Can you work these out from the model? Positions are in its coordinate system, mm. A direction names the side the tool comes from. Round coordinates to 2 decimals unless told otherwise and drop trailing zeros. Order: outer loops, then holes, each group sorted by start corner. A loop starts at its lowest first (then second) coordinate and runs counter-clockwise, first axis right, second up. Notation, with made-up numbers: (46, -14) -> (61, -14) arc R27 cw to (61, 6) -> close; hole circle Ø2 at (38, 77). An arc over 180 degrees is marked (long way). Use a Markdown table: item, result. Add a question column.
Q1. For faces 1 (the face through (0, 1.25, -10)), 2 (the face through (1.3, -1.5, 1.3)), 3 (the face through (-1.08, -2.96, -4.88)), 4 (the face through (2.5, 2.5, 2.5)), which set-ups out of +Z, -Z, +X, -X, +Y, -Y let a thin tool reach every point of the face, with its end or its side?
Q2. I need wall thicknesses on line 1 along Z through (x, y) = (0, -0.1); line 2 along Y through (x, z) = (9, -4.5); line 3 along X through (y, z) = (-4.5, 1.5). Which ranges of each line are inside material? Lowest first, please. Write a range as [from, to].
Q3. If we section it at D-D on z = 10.75: List the corners of the cut face in (x, y) for me, plus the area to 3 significant figures.
Q4. I'm going to push flat-ended pins straight in: pin 1 Ø3 at (x, z) = (-3, 9.5) entering from -Y; pin 2 Ø1 at (x, z) = (5, -7) entering from -Y; pin 3 Ø8 at (x, z) = (0, 0) entering from -Y; pin 4 Ø2.5 at (x, z) = (0, 0) entering from +Y. Where does each tip first touch, or does it pass through?
Q5. If we section it at C-C on y = -0.75: List the corners of the cut face in (x, z) for me.
Q6. If we section it at A-A on z = 0: List the corners of the cut face in (x, y) for me, plus the area to 3 significant figures.
Q7. If we section it at B-B on y = 1.75: List the corners of the cut face in (x, z) for me.
Q8. We'd pull the mould along Z, two halves only. Please class faces 5 (the face through (0, -4, -2)), 6 (the face through (-0.1, -6, -2.2)), 7 (the face through (10.887, 1.51, -5.046)): +Z half, -Z half, draft (parallel to the pull), parting line (faces both ways), or undercut.
```python
from build123d import *

# Parameters (mm, degrees)
CROQUIS1_R              = 12
SALIENTE_EXTRUIR1_DEPTH = 2.5
CROQUIS3_R              = 5
SALIENTE_EXTRUIR2_DEPTH = 6
CROQUIS2_R              = 3.001453564
CORTAR_EXTRUIR1_DEPTH   = 4
CROQUIS4_R              = 1.5
CORTAR_EXTRUIR2_DEPTH   = 8
CROQUIS5_R              = 2
CORTAR_EXTRUIR6_DEPTH   = 4
CROQUIS6_R              = 1.5
CORTAR_EXTRUIR7_DEPTH   = 4
CROQUIS7_R              = 1
CORTAR_EXTRUIR8_DEPTH   = 4
CORTAR_EXTRUIR9_DEPTH   = 1.25


with BuildPart() as part:
    # Croquis1 → Saliente-Extruir1 (new body)
    with BuildSketch(Plane(origin=(0, 0, 0), x_dir=(1, 0, 0), z_dir=(0, 1, 0))):
        Circle(CROQUIS1_R)
    extrude(amount=SALIENTE_EXTRUIR1_DEPTH)

    # Croquis3 → Saliente-Extruir2 (add)
    with BuildSketch(Plane.XZ):
        Circle(CROQUIS3_R)
    extrude(amount=SALIENTE_EXTRUIR2_DEPTH)

    # Croquis2 → Cortar-Extruir1 (cut)
    with BuildSketch(Plane(origin=(0, 2.5, 0), x_dir=(1, 0, 0), z_dir=(0, 1, 0))):
        Circle(CROQUIS2_R)
    extrude(amount=-CORTAR_EXTRUIR1_DEPTH, mode=Mode.SUBTRACT)

    # Croquis4 → Cortar-Extruir2 (cut)
    with BuildSketch(Plane(origin=(0, -1.5, 0), x_dir=(1, 0, 0), z_dir=(0, 1, 0))):
        Circle(CROQUIS4_R)
    extrude(amount=-CORTAR_EXTRUIR2_DEPTH, mode=Mode.SUBTRACT)

    # Croquis5 → Cortar-Extruir6 (cut)
    with BuildSketch(Plane.XZ.offset(6)):
        Circle(CROQUIS5_R)
    extrude(amount=-CORTAR_EXTRUIR6_DEPTH, mode=Mode.SUBTRACT)

    # Croquis6 → Cortar-Extruir7 (cut)
    with BuildSketch(Plane(origin=(0, 2.5, 0), x_dir=(1, 0, 0), z_dir=(0, 1, 0))):
        with Locations((6.363961031, 6.363961031)):
            Circle(CROQUIS6_R)
        with Locations((-6.363961031, -6.363961031)):
            Circle(CROQUIS6_R)
    extrude(amount=-CORTAR_EXTRUIR7_DEPTH, mode=Mode.SUBTRACT)

    # Croquis7 → Cortar-Extruir8 (cut)
    with BuildSketch(Plane.XZ):
        with Locations((8.485281374, 8.485281374)):
            Circle(CROQUIS7_R)
        with Locations((-8.485281374, -8.485281374)):
            Circle(CROQUIS7_R)
    extrude(amount=-CORTAR_EXTRUIR8_DEPTH, mode=Mode.SUBTRACT)

    # Croquis8 → Cortar-Extruir9 (cut)
    with BuildSketch(Plane.XZ):
        with BuildLine():
            ThreePointArc((7.778174593, 7.778174593), (7.485498506, 8.464443516), (7.749325885, 9.162311298))
            ThreePointArc((7.749325885, 9.162311298), (-0.5, 11.989578808), (-8.485281374, 8.485281374))
            add(Edge.make_bspline(
                [(-8.485281374, 8.485281374), (-7.592740334, 8.845120344), (-6.313852411, 9.008442263), (-4.858999126, 8.387047865), (-4.264313018, 7.608507158), (-4.072837383, 6.86756437), (-4.147476561, 6.387348921), (-3.967074672, 6.478559767)],
                knots=[0, 0, 0, 0, 0.492098519, 0.601947317, 0.788100157, 0.955757021, 1, 1, 1, 1], degree=3))
            add(Edge.make_bspline(
                [(7.778174593, 7.778174593), (6.043762471, 8.553284771), (1.93848679, 8.683425804), (-2.11467577, 7.905967318), (-3.967074672, 6.478559767)],
                knots=[0, 0, 0, 0, 0.452400817, 1, 1, 1, 1], degree=3))
        make_face()
        with BuildLine():
            ThreePointArc((-7.749325885, -9.162311298), (0.5, -11.989578808), (8.485281374, -8.485281374))
            add(Edge.make_bspline(
                [(8.485281374, -8.485281374), (7.761300195, -8.818220731), (6.448317824, -9.091275119), (4.851033429, -8.31231131), (4.115527792, -7.425847437), (3.966487119, -6.478710331), (3.548635711, -6.917914395)],
                knots=[0, 0, 0, 0, 0.407620337, 0.622914437, 0.853292729, 1, 1, 1, 1], degree=3))
            add(Edge.make_bspline(
                [(-7.778174593, -7.778174593), (-4.168772685, -9.273462944), (0.223344673, -9.411626111), (3.548635711, -6.917914395)],
                knots=[0, 0, 0, 0, 1, 1, 1, 1], degree=3))
            ThreePointArc((-7.778174593, -7.778174593), (-7.485498506, -8.464443516), (-7.749325885, -9.162311298))
        make_face()
    extrude(amount=-CORTAR_EXTRUIR9_DEPTH, mode=Mode.SUBTRACT)


solid = part.part
```
Answer below:
| question | item | result |
|---|---|---|
| 1 | face 1 | -Z, -Y |
| 1 | face 2 | +Y |
| 1 | face 3 | -Y |
| 1 | face 4 | +Z, -Z, +X, -X, +Y |
| 2 | line 1 | [-5, -3], [3, 5] |
| 2 | line 2 | [0, 2.5] |
| 2 | line 3 | [-4.77, -1.32], [1.32, 4.77] |
| 3 | outline | (-5.33, 1.25) -> (5.33, 1.25) -> (5.33, 2.5) -> (-5.33, 2.5) -> close |
| 3 | area | 13.3 mm² |
| 4 | pin 1 | y = 1.25 |
| 4 | pin 2 | y = 0 |
| 4 | pin 3 | y = -6 |
| 4 | pin 4 | through |
| 5 | outline | circle Ø10 at (0, 0); hole circle Ø6 at (0, 0) |
| 6 | outline | (-12, 0) -> (-5, 0) -> (-5, -6) -> (-2, -6) -> (-2, -2) -> (-1.5, -2) -> (-1.5, -1.5) -> (-3, -1.5) -> (-3, 2.5) -> (-12, 2.5) -> close; (1.5, -2) -> (2, -2) -> (2, -6) -> (5, -6) -> (5, 0) -> (12, 0) -> (12, 2.5) -> (3, 2.5) -> (3, -1.5) -> (1.5, -1.5) -> close |
| 6 | area | 78.5 mm² |
| 7 | outline | (-9.16, -7.75) arc R1 cw to (-7.75, -9.16) arc R12 ccw to (9.16, 7.75) arc R1 cw to (7.75, 9.16) arc R12 ccw to start; hole circle Ø3 at (-6.36, 6.36); hole circle Ø6 at (0, 0); hole circle Ø3 at (6.36, -6.36) |
| 8 | face 5 | undercut |
| 8 | face 6 | draft |
| 8 | face 7 | parting line |
